Could you check a few things on this drawing? It's one solid part, dimensions in mm from its lowest x, y, z. Give positions to 0.01 mm unless a question says otherwise; leave off trailing zeros. Order: outer loops, then holes, each group sorted by start corner. A loop starts at its lowest first (then second) coordinate and runs counter-clockwise, first axis right, second up. Notation, with made-up numbers: (30.5, 85) - (37.5, 85) arc R21 ccw to (37.5, 106) - close; hole circle Ø8 at (61.25, 79). An arc over 180 degrees is marked (long way). Return JSON: item names as keys, results as strings.
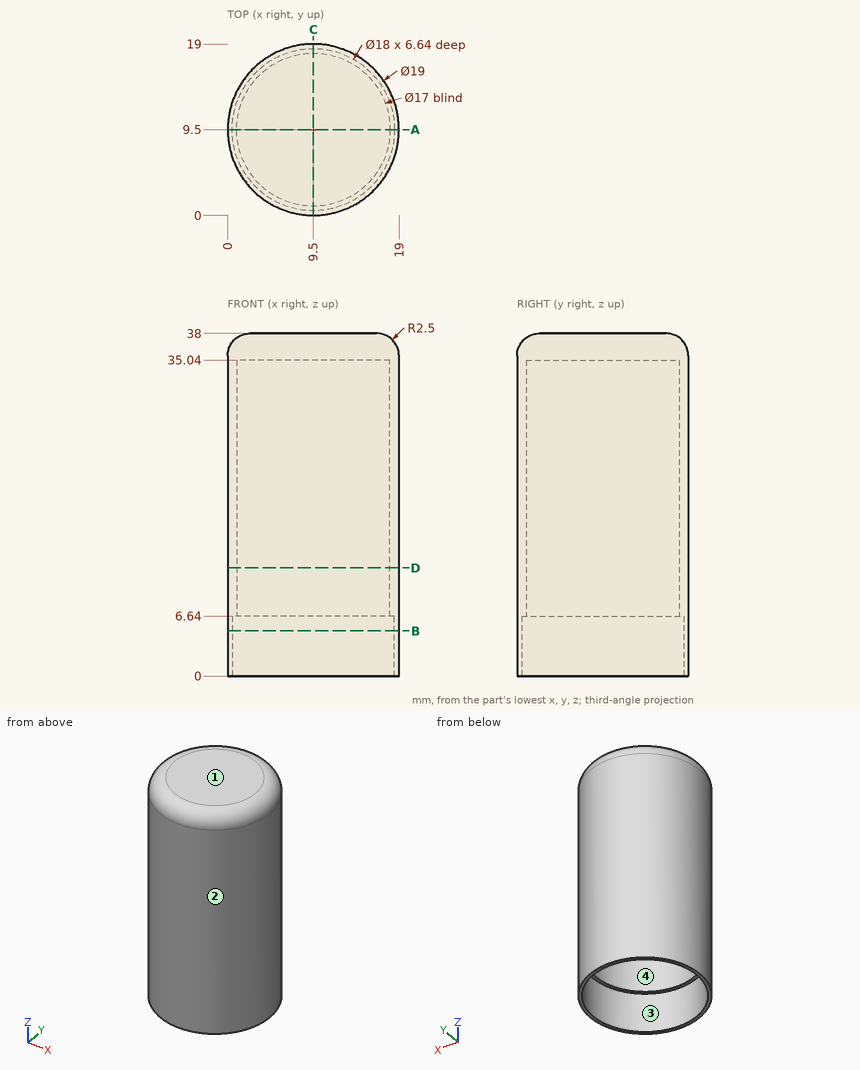
1. Suppose I cut it at A-A (y = 9.5). List the corners of the cut face in (x, z) for me.
Checks:
{"outline": "(0, 0) - (0.5, 0) - (0.5, 6.64) - (1, 6.64) - (1, 35.04) - (18, 35.04) - (18, 6.64) - (18.5, 6.64) - (18.5, 0) - (19, 0) - (19, 35.5) arc R2.5 ccw to (16.5, 38) - (2.5, 38) arc R2.5 ccw to (0, 35.5) - close"}
2. For pin 1 Ø5 at (x, z) = (8, 11.5) entering from -Y; pin 2 Ø3 at (x, y) = (11.5, 16.5) entering from -Z; pin 3 Ø1 at (y, z) = (8.5, 4.5) entering from +X; pin 4 Ø8.5 at (x, y) = (11, 12) entering from -Z, each with a flat end and sliding along its axis, tell me the tip position at first contact or that it passes through.
Checks:
{"pin 1": "y = 0", "pin 2": "z = 6.64", "pin 3": "x = 18.99", "pin 4": "z = 35.04"}
3. If I drill on L1, parallel to X at y = 9.25, z = 33; L2, parallel to Y at x = 9.5, z = 4.5, over which ranges is the centre line in solid material (lowest first)? Write a range as [from, to].
Checks:
{"L1": "[0, 1], [18, 19]", "L2": "[0, 0.5], [18.5, 19]"}
4. Suppose I cut it at B-B (z = 5). List the corners of the cut face in (x, y) for me, plus the area to 3 significant figures.
Checks:
{"outline": "circle Ø19 at (9.5, 9.5); hole circle Ø18 at (9.5, 9.5)", "area": "29.1 mm^2"}
5. Suppose I cut it at D-D (z = 12). List the corners of the cut face in (x, y) for me.
Checks:
{"outline": "circle Ø19 at (9.5, 9.5); hole circle Ø17 at (9.5, 9.5)"}
6. Thinking about a two-plate mould opening in Y: for the marked faces 1, 2, 3 and 4, which applies, +Y half, -Y half, draft (parallel to the pull), parting line (faces both ways), or undercut?
Checks:
{"face 1": "draft", "face 2": "parting line", "face 3": "undercut", "face 4": "undercut"}
